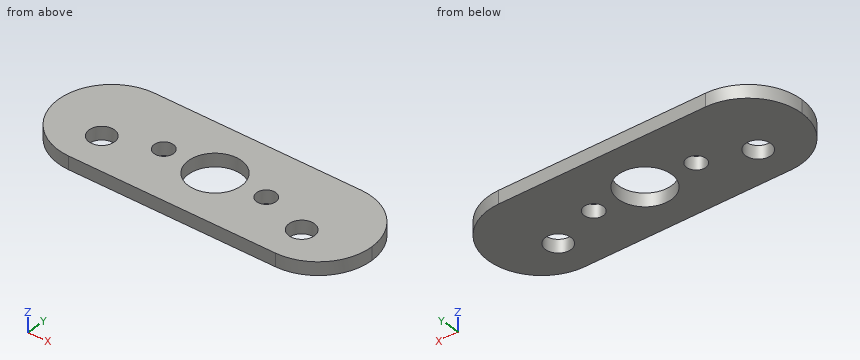
```python
from build123d import *

# Parameters (mm, degrees)
MODEL_R                 = 1.55
MODEL_R_2               = 1.175
MODEL_R_3               = 3.225
SALIENTE_EXTRUIR1_DEPTH = 1.6


with BuildPart() as part:
    # Model → Saliente-Extruir1 (new body)
    with BuildSketch(Plane.XY):
        with BuildLine():
            Line((18.99, -0.000135429), (18.99, 0.019864571))
            ThreePointArc((18.99, 0.019864571), (17.082224275, 4.596089282), (12.5003, 6.490135416))
            ThreePointArc((12.5003, 6.490135429), (12.5, 6.489835429), (12.4997, 6.490135429))
            Line((12.4997, 6.490135429), (0, 6.490135429))
            Line((0, 6.490135429), (-12.4997, 6.490135429))
            ThreePointArc((-12.4997, 6.490135429), (-12.499999997, 6.489835429), (-12.5003, 6.490135422))
            ThreePointArc((-12.5003, 6.490135422), (-17.085798512, 4.592642615), (-18.990142559, 0.009985166))
            Line((-18.990142559, 0.009985166), (-18.990142559, -0.010014834))
            ThreePointArc((-18.990142559, -0.010014834), (-17.085798512, -4.592672284), (-12.5003, -6.490165091))
            ThreePointArc((-12.5003, -6.490165091), (-12.499999997, -6.489865098), (-12.4997, -6.490165098))
            Line((-12.4997, -6.490165098), (12.4997, -6.490135429))
            ThreePointArc((12.4997, -6.490135429), (12.5, -6.489835429), (12.5003, -6.490135429))
            ThreePointArc((12.5003, -6.490135415), (17.089185065, -4.589108362), (18.99, -0.000135429))
        make_face()
        with Locations((-12.1, -2)):
            Circle(MODEL_R, mode=Mode.SUBTRACT)
        with Locations((12.1, -2)):
            Circle(MODEL_R, mode=Mode.SUBTRACT)
        with Locations((-6.2, 0)):
            Circle(MODEL_R_2, mode=Mode.SUBTRACT)
        Circle(MODEL_R_3, mode=Mode.SUBTRACT)
        with Locations((6.2, 0)):
            Circle(MODEL_R_2, mode=Mode.SUBTRACT)
    extrude(amount=SALIENTE_EXTRUIR1_DEPTH)


solid = part.part
```
CAD build for the part. Positions are in the model's coordinates, mm. Round coordinates to 2 decimals unless told otherwise and drop trailing zeros. Loops run counter-clockwise (first coordinate to the right, second up) from the corner with the lowest first, then second, coordinate; pieces in that order, holes last. Notation, with made-up numbers: M 21,-30.5 L 41,-30.5 A15 cw 41,-4.5 Z; hole C -6.5,-37 d10. An arc over 180 degrees is marked long. Return JSON: item names as keys, results as strings. Group by question number.
(1) Saw through at D-D, the plane y = 2. List the corners of the cut face in (x, z).
(2) Saw through at A-A, the plane z = 0.45. Give the number of separate pieces and of enclosed holes in the cut face, and give its area (3 significant figures).
(3) Saw through at B-B, the plane x = 6.2. List the corners of the cut face in (y, z) (3 decimals), and give its area (3 significant figures).
(4) Saw through at C-C, the plane y = -2. List the corners of the cut face in (x, z), and give its area (3 significant figures).
(5) Wall check: probe 1 along X at (y, z) = (-0.25, 0.4); probe 2 along Y at (x, z) = (-6.2, 0.65) (3 decimals); probe 3 along X at (y, z) = (-1, 0.65). Give the ranges that are in metal, low to high. Write a range as [from, to].
Answer list:
{
 "1": {"outline": "M -18.67,0 L -2.53,0 L -2.53,1.6 L -18.67,1.6 Z; M 2.53,0 L 18.67,0 L 18.67,1.6 L 2.53,1.6 Z"},
 "2": {"separate pieces": "1", "enclosed holes": "5", "area": "400 mm2"},
 "3": {"outline": "M -6.49,0 L -1.175,0 L -1.175,1.6 L -6.49,1.6 Z; M 1.175,0 L 6.49,0 L 6.49,1.6 L 1.175,1.6 Z", "area": "17.0 mm2"},
 "4": {"outline": "M -18.67,0 L -13.65,0 L -13.65,1.6 L -18.67,1.6 Z; M -10.55,0 L -2.53,0 L -2.53,1.6 L -10.55,1.6 Z; M 2.53,0 L 10.55,0 L 10.55,1.6 L 2.53,1.6 Z; M 13.65,0 L 18.67,0 L 18.67,1.6 L 13.65,1.6 Z", "area": "41.7 mm2"},
 "5": {"probe 1": "[-18.99, -7.35], [-5.05, -3.22], [3.22, 5.05], [7.35, 18.99]", "probe 2": "[-6.49, -1.175], [1.175, 6.49]", "probe 3": "[-18.91, -13.28], [-10.92, -6.82], [-5.58, -3.07], [3.07, 5.58], [6.82, 10.92], [13.28, 18.91]"}
}
